from build123d import *

# Parameters (mm, degrees)
LID_BLOCK_START      = 48
SKETCH1_W            = 27
SKETCH1_H            = 27
LID_BLOCK_DEPTH      = 14.5
MAGNET_EAR_START     = 48
SKETCH2_W            = 30
SKETCH2_H            = 16
MAGNET_EAR_DEPTH     = 14.5
SKIRT_RECESS_START   = 48
SKETCH3_W            = 23.4
SKETCH3_H            = 23.4
SKIRT_RECESS_DEPTH   = 6
CUVETTE_CAVITY_START = 54
SKETCH4_W            = 15
SKETCH4_H            = 15
CUVETTE_CAVITY_DEPTH = 5.5
MAGNET_POCKET_START  = 48
SKETCH5_W            = 27.4
SKETCH5_H            = 14.4
MAGNET_POCKET_DEPTH  = 8.2


with BuildPart() as part:
    # Sketch1 → Lid_Block (new body)
    with BuildSketch(Plane(origin=(0, 0, 0), x_dir=(1, 0, 0), z_dir=(0, 1, 0)).offset(LID_BLOCK_START)):
        Rectangle(SKETCH1_W, SKETCH1_H)
    extrude(amount=LID_BLOCK_DEPTH)

    # Sketch2 → Magnet_Ear (add)
    with BuildSketch(Plane(origin=(0, 0, 0), x_dir=(1, 0, 0), z_dir=(0, 1, 0)).offset(MAGNET_EAR_START)):
        with Locations((0, -21.5)):
            Rectangle(SKETCH2_W, SKETCH2_H)
    extrude(amount=MAGNET_EAR_DEPTH)

    # Sketch3 → Skirt_Recess (cut)
    with BuildSketch(Plane(origin=(0, 0, 0), x_dir=(1, 0, 0), z_dir=(0, 1, 0)).offset(SKIRT_RECESS_START)):
        Rectangle(SKETCH3_W, SKETCH3_H)
    extrude(amount=SKIRT_RECESS_DEPTH, mode=Mode.SUBTRACT)

    # Sketch4 → Cuvette_Cavity (cut)
    with BuildSketch(Plane(origin=(0, 0, 0), x_dir=(1, 0, 0), z_dir=(0, 1, 0)).offset(CUVETTE_CAVITY_START)):
        Rectangle(SKETCH4_W, SKETCH4_H)
    extrude(amount=CUVETTE_CAVITY_DEPTH, mode=Mode.SUBTRACT)

    # Sketch5 → Magnet_Pocket (cut)
    with BuildSketch(Plane(origin=(0, 0, 0), x_dir=(1, 0, 0), z_dir=(0, 1, 0)).offset(MAGNET_POCKET_START)):
        with Locations((0, -21.5)):
            Rectangle(SKETCH5_W, SKETCH5_H)
    extrude(amount=MAGNET_POCKET_DEPTH, mode=Mode.SUBTRACT)


solid = part.part
For this review, take the finished solid that the model builds, in its own axes (mm). A direction names the side the tool comes from. Give positions to 0.01 mm unless a question says otherwise; leave off trailing zeros. Loops run counter-clockwise (first coordinate to the right, second up) from the corner with the lowest first, then second, coordinate; pieces in that order, holes last. Notation, with made-up numbers: (-23.5, -18) - (-5.5, -18) arc R21 cw to (-5.5, 3) - close; hole circle Ø10 at (-16, 8). An arc over 180 degrees is marked (long way). Write each question's results on one line, items separated by ' | '.
(1) For pin 1 Ø8 at (x, z) = (1.5, 10) entering from -Y; pin 2 Ø3 at (y, z) = (56.5, 7.5) entering from -X; pin 3 Ø1.6 at (y, z) = (55.5, -1) entering from +X; pin 4 Ø1 at (x, z) = (4.5, 0.5) entering from -Y, all flat-tipped, find the tip position at first contact; note any pin that passes through.
Conclusion:
pin 1: y = 48 | pin 2: x = -13.5 | pin 3: x = 13.5 | pin 4: y = 59.5
(2) Take a section at A-A (z = -1.5). Give the boundary of the cut face in (x, y).
Conclusion:
outline: (-13.5, 48) - (-11.7, 48) - (-11.7, 54) - (-7.5, 54) - (-7.5, 59.5) - (7.5, 59.5) - (7.5, 54) - (11.7, 54) - (11.7, 48) - (13.5, 48) - (13.5, 62.5) - (-13.5, 62.5) - close
(3) Draft analysis for pull direction X (two halves, no side actions). For faces 1 (the flat face through (-15, 55, 22)), 2 (the flat face through (-13.7, 52, 22)), 3 (the flat face through (-14, 55, 13.5)), state which applies: +X half, -X half, draft (parallel to the pull), parting line (faces both ways), or undercut.
Conclusion:
face 1: -X half | face 2: undercut | face 3: draft
(4) Take a section at B-B (y = 52.25). Give the boundary of the cut face in (x, z).
Conclusion:
outline: (-15, 13.5) - (-13.5, 13.5) - (-13.5, -13.5) - (13.5, -13.5) - (13.5, 13.5) - (15, 13.5) - (15, 29.5) - (-15, 29.5) - close; hole (-13.7, 14.3) - (13.7, 14.3) - (13.7, 28.7) - (-13.7, 28.7) - close; hole (-11.7, -11.7) - (11.7, -11.7) - (11.7, 11.7) - (-11.7, 11.7) - close
(5) Take a section at D-D (y = 57). Give the boundary of the cut face in (x, z).
Conclusion:
outline: (-15, 13.5) - (-13.5, 13.5) - (-13.5, -13.5) - (13.5, -13.5) - (13.5, 13.5) - (15, 13.5) - (15, 29.5) - (-15, 29.5) - close; hole (-7.5, -7.5) - (7.5, -7.5) - (7.5, 7.5) - (-7.5, 7.5) - close
(6) For line 1 along Z through (x, y) = (-11.25, 49.5); line 2 along X through (y, z) = (53.25, 27.5); line 3 along Z through (x, y) = (0, 58), list the stretches that pass through material, from the lowest coordinate up.
Conclusion:
line 1: -13.5 to -11.7, 11.7 to 14.3, 28.7 to 29.5 | line 2: -15 to -13.7, 13.7 to 15 | line 3: -13.5 to -7.5, 7.5 to 29.5
(7) Take a section at C-C (x = -4.5). Give the boundary of the cut face in (y, z).
Conclusion:
outline: (48, -13.5) - (62.5, -13.5) - (62.5, 29.5) - (48, 29.5) - (48, 28.7) - (56.2, 28.7) - (56.2, 14.3) - (48, 14.3) - (48, 11.7) - (54, 11.7) - (54, 7.5) - (59.5, 7.5) - (59.5, -7.5) - (54, -7.5) - (54, -11.7) - (48, -11.7) - close
(8) For faces 4 (the flat face through (-11.7, 51, 0)), 5 (the flat face through (0, 55, -13.5)), 6 (the flat face through (13.5, 55, 0)), 7 (the flat face through (-13.5, 55, 0)), list the 3-axis set-ups (+Z, -Z, +X, -X, +Y, -Y) from which the entire face can be reached by the end or side of a thin tool; tool diameter is ignored.
Conclusion:
face 4: -Y | face 5: -Z, +X, -X, +Y, -Y | face 6: -Z, +X, +Y, -Y | face 7: -Z, -X, +Y, -Y
